Source: three-view drawing plus pictorial views. Frame: mm from the lowest corner of the part. Give positions to 0.01 mm unless a question says otherwise; leave off trailing zeros. Loops run counter-clockwise (first coordinate to the right, second up) from the corner with the lowest first, then second, coordinate; pieces in that order, holes last. Notation, with made-up numbers: M 52.25,67 L 81.25,67 A20 cw 81.25,104 Z; hole C 28,-25 d3. An arc over 180 degrees is marked long. Answer as a JSON object with one key per item and string values. Group by question number.
1) Section query C-C on y = 5.25. Return loops of the section in (x, z), plus the area to 3 significant figures.
2) First-contact query: P1, Ø1.5, axis at x = 12.7, z = 3.5, coming from the +Y side; P2, Ø6, axis at x = 18.5, z = 13.5, coming from the -Y side; P3, Ø4, axis at y = 2.5, z = 14.5, coming from the -X side; P4, Ø2, axis at x = 32.7, z = 23.5, coming from the +Y side. Flat tips, straight axial feed; report the tip coordinate or a pass-through.
3) Ray query, L1, parallel to X at y = 11.9, z = 23.5; L2, parallel to Z at x = 32.7, y = 10.7; L3, parallel to Z at x = 38.5, y = 3.5. Return the intervals inside material, ascending.
4) Section query D-D on z = 14. Return loops of the section in (x, y).
5) Section query A-A on y = 3. Return loops of the section in (x, z).
6) Section query B-B on x = 27. Return loops of the section in (y, z), plus the area to 3 significant figures.
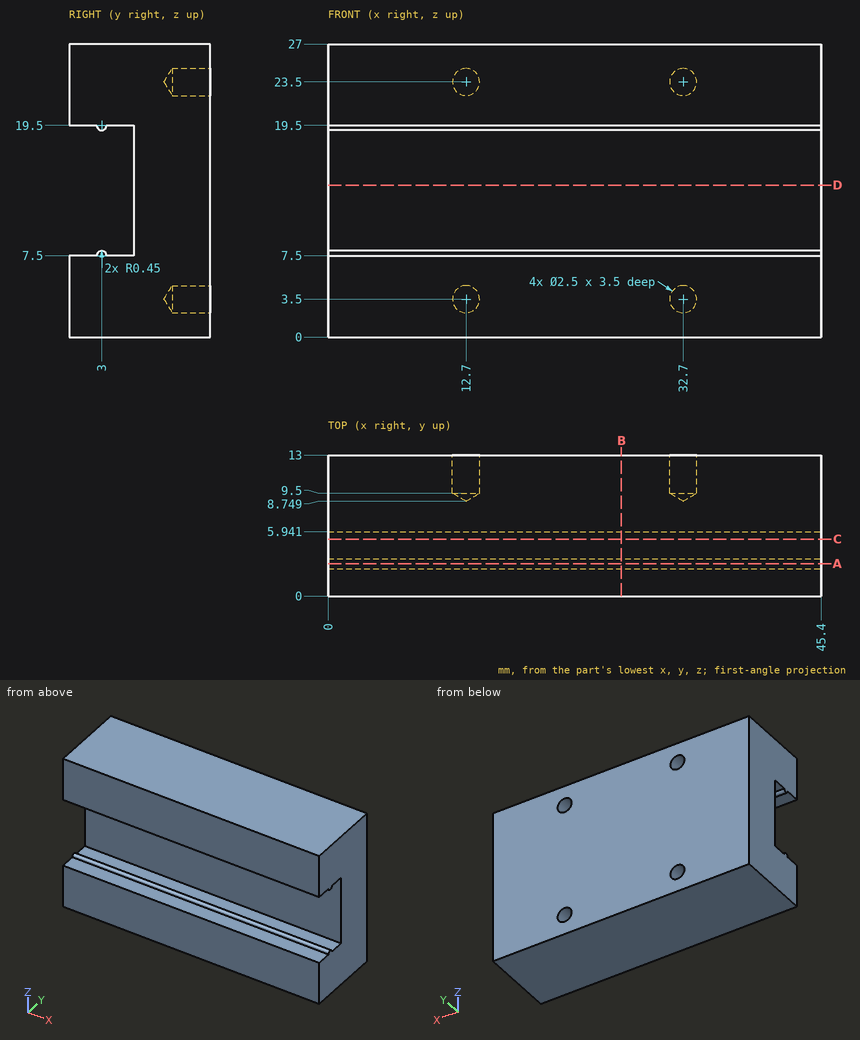
Output:
{
 "1": {"outline": "M 0,0 L 45.4,0 L 45.4,7.5 L 0,7.5 Z; M 0,19.5 L 45.4,19.5 L 45.4,27 L 0,27 Z", "area": "681 mm^2"},
 "2": {"P1": "stops at y = 9.2", "P2": "stops at y = 5.94", "P3": "passes through", "P4": "stops at y = 9.35"},
 "3": {"L1": "x = 0 to 11.45, 13.95 to 31.45, 33.95 to 45.4", "L2": "z = 0 to 2.25, 4.75 to 22.25, 24.75 to 27", "L3": "z = 0 to 7.5, 19.5 to 27"},
 "4": {"outline": "M 0,5.94 L 45.4,5.94 L 45.4,13 L 0,13 Z"},
 "5": {"outline": "M 0,0 L 45.4,0 L 45.4,7.95 L 0,7.95 Z; M 0,19.05 L 45.4,19.05 L 45.4,27 L 0,27 Z"},
 "6": {"outline": "M 0,0 L 13,0 L 13,27 L 0,27 L 0,19.5 L 2.55,19.5 A0.45 ccw 3.45,19.5 L 5.94,19.5 L 5.94,7.5 L 3.45,7.5 A0.45 ccw 2.55,7.5 L 0,7.5 Z", "area": "280 mm^2"}
}
